Autodesk Inventor part; units mm, degrees
ref_plane "YZ Plane" through (0, 0, 0) normal (1, 0, 0) x (0, 1, 0)
ref_plane "XZ Plane" through (0, 0, 0) normal (0, 1, 0) x (-1, 0, 0)
ref_plane "XY Plane" through (0, 0, 0) normal (0, 0, 1) x (1, 0, 0)
sketch "Sketch1" plane through (0, 0, 0) normal (0, 1, 0) x (-1, 0, 0)
  line L0 (0, 0) -> (-25.4, 0)
  line L1 (-25.4, 0) -> (-25.4, -25.4)
  line L2 (-25.4, -25.4) -> (0, -25.4)
  line L3 (0, -25.4) -> (0, 0)
  dimension "d0" = 25.4
extrude "Extrusion1" add sketch "Sketch1" along normal blind 6.35
sketch "Sketch2" plane through (0, 6.35, 0) normal (0, 1, 0) x (1, 0, 0)
  circle A0 centre (8.4667, 13.97) radius 0.635
  circle A1 centre (16.9333, 13.97) radius 0.635
  circle A2 centre (16.9333, 11.43) radius 0.635
  circle A3 centre (8.4667, 11.43) radius 0.635
  line L0 (25.4, 0) -> (25.4, 25.4)
  line L1 (0, 0) -> (25.4, 0)
  dimension "d3" = 8.4667
  dimension "d4" = 8.4667
  dimension "d5" = 2.54
  dimension "d6" = 1.27
  dimension "d7" = 11.43
extrude "Extrusion2" cut sketch "Sketch2" against normal blind 6.35
sketch "Sketch4" plane through (0, 0, 0) normal (0, -1, 0) x (1, 0, 0)
  line L0 (25.4, -25.4) -> (0, -25.4)
  arc A0 (9.525, -25.4) -> (15.875, -25.4) centre (12.7, -28.575) ccw
  line L1 (15.875, -25.4) -> (9.525, -25.4)
  point P0 (0, 0)
  dimension "d10" = 90
  dimension "d11" = 6.35
  dimension "d12" = 9.525
extrude "Extrusion3" add sketch "Sketch4" against normal blind 3.175
sketch "Sketch6" plane through (0, 0, 0) normal (0, -1, 0) x (1, 0, 0)
  line L0 (25.4, 0) -> (25.4, -25.4)
  arc A0 (25.4, -9.525) -> (25.4, -15.875) centre (22.225, -12.7) ccw
  line L1 (25.4, -15.875) -> (25.4, -9.525)
  point P0 (0, 0)
  dimension "d21" = 6.35
  dimension "d22" = 90
  dimension "d23" = 9.525
extrude "Extrusion5" cut sketch "Sketch6" against normal blind 3.175
equation "\"d1\" = 0.25 * d0"
equation "\"d3\" = 0.333333 * d0"
equation "\"d4\" = d3"
equation "\"d8\" = 0.25 * d0"
equation "\"d11\" = 0.25 * d0"
equation "\"d12\" = 0.375 * d0"
equation "\"d13\" = 0.5 * d1"
equation "\"d21\" = 0.25 * d0"
equation "\"d23\" = 0.375 * d0"
equation "\"d24\" = 0.5 * d1"
properties part number "pieceBase"
Design review of the part built by this model. Coordinates are the model's own, in mm. A direction names the side the tool comes from. Coordinates: 2 decimals unless noted, no trailing zeros. Loops run counter-clockwise (first coordinate to the right, second up) from the corner with the lowest first, then second, coordinate; pieces in that order, holes last.
Q1. To check wall thickness, follow line 1 (X direction, y = 4.75, z = -11.43); line 2 (X direction, y = 3, z = -11.43); line 3 (Z direction, x = 17.5, y = 1). State the ranges of each line that lie inside material, in increasing order.
Reported:
line 1: x = 0 to 7.83, 9.1 to 16.3, 17.57 to 25.4
line 2: x = 0 to 7.83, 9.1 to 16.3, 17.57 to 17.92
line 3: z = -25.4 to -14.26, -13.68 to -11.72, -11.14 to 0
Q2. For pin 1 (4 mm diameter, centred on x = 23, z = -11.5, fed in from -Y) (3 decimals), flat-tipped, find the tip position at first contact; note if it passes through.
Reported:
pin 1: stops at y = 3.175
Q3. We need section C-C on y = 0.5. State the section outline as (x, z) points (3 decimals), and give its area (3 significant figures).
Reported:
outline: (0, -25.4) - (9.525, -25.4) arc R4.49 ccw (long way) to (15.875, -25.4) - (25.4, -25.4) - (25.4, -15.875) arc R4.49 cw (long way) to (25.4, -9.525) - (25.4, 0) - (0, 0) - close; hole circle Ø1.27 at (8.467, -13.97); hole circle Ø1.27 at (8.467, -11.43); hole circle Ø1.27 at (16.933, -13.97); hole circle Ø1.27 at (16.933, -11.43)
area: 640 mm2
Q4. We need section B-B on x = 12.7. State the section outline as (y, z) points (3 decimals), and give its area (3 significant figures).
Reported:
outline: (0, -33.065) - (3.175, -33.065) - (3.175, -25.4) - (6.35, -25.4) - (6.35, 0) - (0, 0) - close
area: 186 mm2
Q5. We need section A-A on z = -12.7. State the section outline as (x, y) points (3 decimals), and give its area (3 significant figures).
Reported:
outline: (0, 0) - (17.735, 0) - (17.735, 3.175) - (25.4, 3.175) - (25.4, 6.35) - (0, 6.35) - close
area: 137 mm2
Q6. The part is to be moulded in two halves that separate along Z. For faces 1 (the face through (13, 3, 0)), 2 (the face through (16.3, 3.2, -14)), 3 (the face through (25.4, 4, -13)), say which applies: +Z half, -Z half, draft (parallel to the pull), parting line (faces both ways), or undercut.
Reported:
face 1: +Z half
face 2: undercut
face 3: draft
Q7. Tool access review of faces 4 (the face through (17.737, 1.565, -12.552)), 5 (the face through (13, 0, -13)), 6 (the face through (13, 3.175, -29)): name each direction out of +Z, -Z, +X, -X, +Y, -Y from which nothing blocks a thin tool from reaching the whole face with its end or side.
Reported:
face 4: -Y
face 5: +Z, -Z, +X, -X, -Y
face 6: -Z, +X, -X, +Y
Q8. We need section D-D on x = 19.25. State the section outline as (y, z) points (3 decimals), and give its area (3 significant figures).
Reported:
outline: (0, -25.4) - (6.35, -25.4) - (6.35, 0) - (0, 0) - (0, -9.337) - (3.175, -9.337) - (3.175, -16.063) - (0, -16.063) - close
area: 140 mm2
